Source: three-view drawing plus pictorial views. Frame: mm from the lowest corner of the part. A direction names the side the tool comes from. Give positions to 0.01 mm unless a question says otherwise; leave off trailing zeros. Order: outer loops, then holes, each group sorted by start corner. A loop starts at its lowest first (then second) coordinate and runs counter-clockwise, first axis right, second up.
1) Section A-A, the plane z = 7.75. Return loops of the section in (x, y) (1 decimal).
2) Material intervals for line 1 (Y direction, x = 2.25, z = 10.5) (1 decimal); line 2 (X direction, y = 0.8, z = 8.75) (1 decimal), sorted ascending.
3) Access query for the marked faces 1, 2, 3 and 4. Directions: +Z, -Z, +X, -X, +Y, -Y. A direction counts if a zero-diameter tool reaches every point of the face in a straight line with its end or side. Return the directions, or none.
4) First-contact query: P1, Ø2, axis at y = 1, z = 6.5, coming from the -X side; P2, Ø3, axis at x = 4, y = 1.5, coming from the -Z side; P3, Ø3, axis at y = 2.5, z = 8.5, coming from the +X side; P4, Ø1.8, axis at x = 2.5, z = 8, coming from the +Y side. Flat tips, straight axial feed; report the tip coordinate or a pass-through.
5) Section C-C, the plane y = 3.6. Return loops of the section in (x, z) (1 decimal).
6) Draft query along X for the marked faces 5, 6, 7 and 8. Return one class per face: released by +X, released by -X, zero draft, split by the parting line, or undercut.
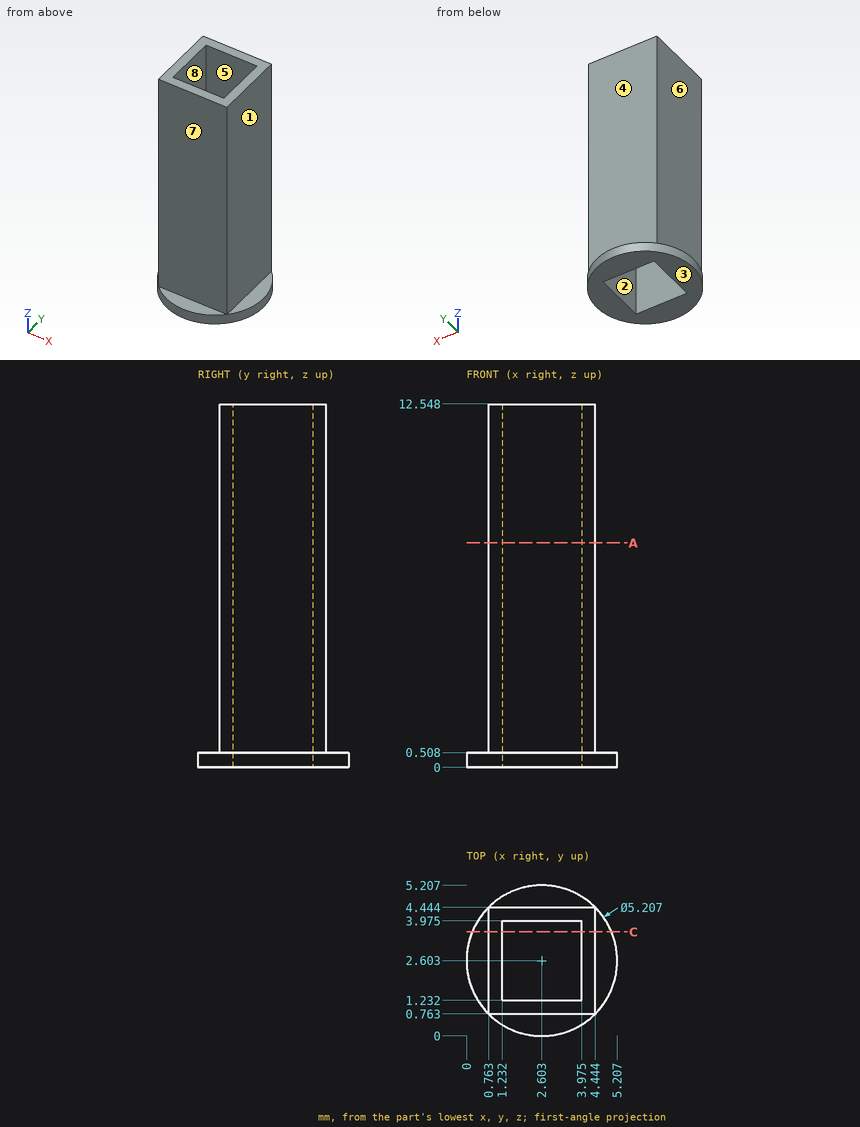
From the geometry:
1. outline: (0.8, 0.8) - (4.4, 0.8) - (4.4, 4.4) - (0.8, 4.4) - close; hole (1.2, 1.2) - (4, 1.2) - (4, 4) - (1.2, 4) - close
2. line 1: y = 0.8 to 1.2, 4 to 4.4
2. line 2: x = 0.8 to 4.4
3. face 1: +Z, +X, +Y, -Y
3. face 2: +Z, -Z
3. face 3: -Z, +X, -X, +Y, -Y
3. face 4: +Z, +X, -X, +Y
4. P1: stops at x = 0.76
4. P2: stops at z = 0
4. P3: stops at x = 4.44
4. P4: stops at y = 4.44
5. outline: (0.2, 0) - (1.2, 0) - (1.2, 12.5) - (0.8, 12.5) - (0.8, 0.5) - (0.2, 0.5) - close; (4, 0) - (5, 0) - (5, 0.5) - (4.4, 0.5) - (4.4, 12.5) - (4, 12.5) - close
6. face 5: undercut
6. face 6: released by -X
6. face 7: zero draft
6. face 8: undercut
